from build123d import *

# Parameters (mm, degrees)
SKETCH2_R           = 157
BOSS_EXTRUDE1_DEPTH = 10
BOSS_EXTRUDE2_START = 15
BOSS_EXTRUDE2_DEPTH = 15
SKETCH4_R           = 25
CUT_EXTRUDE1_DEPTH  = 223.537637266
SKETCH5_R           = 2.6
CUT_EXTRUDE2_DEPTH  = 224.434554176
CIRPATTERN1_COUNT   = 4


with BuildPart() as part:
    # Sketch2 → Boss-Extrude1 (new body)
    with BuildSketch(Plane(origin=(0, 0, 0), x_dir=(1, 0, 0), z_dir=(0, 1, 0))):
        with Locations(Location((0, 0, 0), (0, 0, 270))):
            Circle(SKETCH2_R)
    extrude(amount=-BOSS_EXTRUDE1_DEPTH)

    # Sketch3 → Boss-Extrude2 (add)
    with BuildSketch(Plane(origin=(0, 0, 0), x_dir=(1, 0, 0), z_dir=(0, 1, 0)).offset(BOSS_EXTRUDE2_START)):
        with BuildLine():
            ThreePointArc((157, 0), (0, 157), (-157, 0))
            Line((-157, 0), (-147, 0))
            ThreePointArc((-147, 0), (0, 147), (147, 0))
            Line((147, 0), (157, 0))
        make_face()
    extrude(amount=-BOSS_EXTRUDE2_DEPTH)

    # Sketch4 → Cut-Extrude1 (cut, through all)
    with BuildSketch(Plane(origin=(0, 0, 0), x_dir=(1, 0, 0), z_dir=(0, 1, 0))):
        with Locations(Location((0, 0, 0), (0, 0, 270))):
            Circle(SKETCH4_R)
    extrude(amount=-CUT_EXTRUDE1_DEPTH, mode=Mode.SUBTRACT)

    # Sketch5 → Cut-Extrude2 (cut, through all)
    with BuildSketch(Plane.XZ.offset(10)):
        with Locations(Location((0, 45, 0), (0, 0, 270))):
            Circle(SKETCH5_R)
    cut_extrude2 = extrude(amount=-CUT_EXTRUDE2_DEPTH, mode=Mode.SUBTRACT)

    # CirPattern1: Cut-Extrude2 ×4 about axis
    cirpattern1_axis = Axis((0, 0, 0), (0, 1, 0))
    for i in range(1, CIRPATTERN1_COUNT):
        add(cut_extrude2.rotate(cirpattern1_axis, i * 360 / CIRPATTERN1_COUNT), mode=Mode.SUBTRACT)


solid = part.part
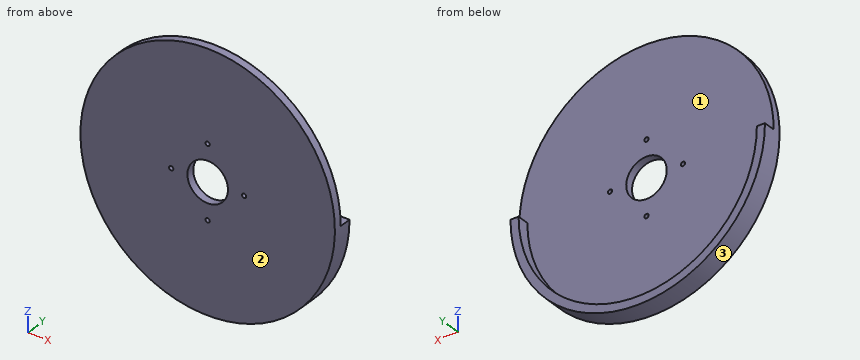
Could you check a few things on this model? Use its own coordinates, in mm. Face numbers are marked on the shaded views. Give positions to 0.01 mm unless a question says otherwise; leave off trailing zeros. Write each loop counter-clockwise with the first axis right and the second up, starting at its lowest first coordinate (ties: lowest second). Pieces come first, ordered by that corner, then holes. Notation, with made-up numbers: (84, 28.5) -> (143, 28.5) arc R8 cw to (143, 42.5) -> close; hole circle Ø6 at (-21.75, -0.5). An arc over 180 degrees is marked (long way). Write each question's results on one line, items separated by ' | '. Start each with the question number.
Q1. I need wall thicknesses on probe 1 along Y at (x, z) = (-98.5, -13.5); probe 2 along Z at (x, y) = (45, -4.25). Which ranges of each line are inside material? Lowest first, please.
Q2. We'd pull the mould along X, two halves only. Please class the marked faces 1, 2 and 3: +X half, -X half, draft (parallel to the pull), parting line (faces both ways), or undercut.
Q3. Suppose I cut it at A-A, the plane y = -5.5. List the corners of the cut face in (x, z) for me.
Q4. Suppose I cut it at B-B, the plane z = -20. List the corners of the cut face in (x, y) for me.
Q5. I'm going to push flat-ended pins straight in: pin 1 Ø1.5 at (x, z) = (-62, -23) entering from +Y; pin 2 Ø7 at (x, z) = (45, 0) entering from -Y; pin 3 Ø8 at (x, y) = (-153.5, 7) entering from +Z; pin 4 Ø10 at (y, z) = (-4, 76) entering from +X. Where does each tip first touch, or does it pass through?
Q6. Suppose I cut it at D-D, the plane x = -37. List the corners of the cut face in (y, z) for me, and give its area (3 significant figures).
Q7. Suppose I cut it at C-C, the plane z = -138. List the corners of the cut face in (x, y) for me.
Outcome:
1) probe 1: -10 to 0 | probe 2: -150.41 to -2.6, 2.6 to 150.41
2) face 1: undercut | face 2: draft | face 3: parting line
3) outline: circle Ø314 at (0, 0); hole circle Ø5.2 at (-45, 0); hole circle Ø50 at (0, 0); hole circle Ø5.2 at (0, -45); hole circle Ø5.2 at (0, 45); hole circle Ø5.2 at (45, 0)
4) outline: (-155.72, -10) -> (-15, -10) -> (-15, 0) -> (-145.63, 0) -> (-145.63, 15) -> (-155.72, 15) -> close; (15, -10) -> (155.72, -10) -> (155.72, 15) -> (145.63, 15) -> (145.63, 0) -> (15, 0) -> close
5) pin 1: y = 0 | pin 2: y = -10 | pin 3: z = 0 | pin 4: x = 140.03
6) outline: (-10, -152.58) -> (15, -152.58) -> (15, -142.27) -> (0, -142.27) -> (0, 152.58) -> (-10, 152.58) -> close | area: 3,210 mm2
7) outline: (-74.87, -10) -> (74.87, -10) -> (74.87, 15) -> (50.65, 15) -> (50.65, 0) -> (-50.65, 0) -> (-50.65, 15) -> (-74.87, 15) -> close
